from build123d import *

# Parameters (mm, degrees)
SKETCH1_W           = 100
SKETCH1_H           = 20
BOSS_EXTRUDE1_DEPTH = 3
SKETCH2_R           = 4
SKETCH2_R_2         = 1.9
SKETCH2_R_3         = 3
SKETCH2_R_4         = 5
BOSS_EXTRUDE2_DEPTH = 14.25
CHAMFER1_SIZE       = 3
CHAMFER2_SIZE       = 3
CHAMFER3_SIZE       = 3
SKETCH14_R          = 4
SKETCH14_R_2        = 1.8
SKETCH14_R_3        = 5
SKETCH14_R_4        = 6
BOSS_EXTRUDE3_DEPTH = 15
CHAMFER4_SIZE       = 7
CUT_EXTRUDE2_START  = 12
CUT_EXTRUDE2_DEPTH  = 2.4
LPATTERN2_COUNT     = 3
LPATTERN2_PITCH     = 15


with BuildPart() as part:
    # Sketch1 → Boss-Extrude1 (new body)
    with BuildSketch(Plane(origin=(0, 0, 0), x_dir=(1, 0, 0), z_dir=(0, 1, 0))):
        Rectangle(SKETCH1_W, SKETCH1_H)
    extrude(amount=BOSS_EXTRUDE1_DEPTH)

    # Sketch2 → Boss-Extrude2 (add)
    # profile 1 of 3: a face of its own
    with BuildSketch(Plane(origin=(0, 3, 0), x_dir=(1, 0, 0), z_dir=(0, 1, 0))):
        with Locations(Location((-25, 0, 0), (0, 0, 90))):
            Circle(SKETCH2_R)
        with Locations(Location((-25, 0, 0), (0, 0, 90))):
            Circle(SKETCH2_R_2, mode=Mode.SUBTRACT)
    # profile 2 of 3: a face of its own
    with BuildSketch(Plane(origin=(0, 3, 0), x_dir=(1, 0, 0), z_dir=(0, 1, 0))):
        with Locations(Location((-40, 0, 0), (0, 0, 90))):
            Circle(SKETCH2_R_3)
        with Locations(Location((-40, 0, 0), (0, 0, 90))):
            Circle(SKETCH2_R_2, mode=Mode.SUBTRACT)
    # profile 3 of 3: a face of its own
    with BuildSketch(Plane(origin=(0, 3, 0), x_dir=(1, 0, 0), z_dir=(0, 1, 0))):
        with Locations(Location((-10, 0, 0), (0, 0, 90))):
            Circle(SKETCH2_R_4)
        with Locations(Location((-10, 0, 0), (0, 0, 90))):
            Circle(SKETCH2_R_2, mode=Mode.SUBTRACT)
    extrude(amount=BOSS_EXTRUDE2_DEPTH)

    # Chamfer1
    chamfer1_edges = [part.edges().sort_by_distance(p)[0] for p in [
        (-40, 3, 3),
    ]]
    chamfer(chamfer1_edges, length=CHAMFER1_SIZE)

    # Chamfer2
    chamfer2_edges = [part.edges().sort_by_distance(p)[0] for p in [
        (-25, 3, 4),
    ]]
    chamfer(chamfer2_edges, length=CHAMFER2_SIZE)

    # Chamfer3
    chamfer3_edges = [part.edges().sort_by_distance(p)[0] for p in [
        (-10, 3, 5),
    ]]
    chamfer(chamfer3_edges, length=CHAMFER3_SIZE - 0.0001)  # a hair under: the kernel refuses the full size

    # Sketch14 → Boss-Extrude3 (add)
    # profile 1 of 3: a face of its own
    with BuildSketch(Plane(origin=(0, 3, 0), x_dir=(1, 0, 0), z_dir=(0, 1, 0))):
        with Locations(Location((10, 0, 0), (0, 0, 90))):
            Circle(SKETCH14_R)
        with Locations(Location((10, 0, 0), (0, 0, 270))):
            Circle(SKETCH14_R_2, mode=Mode.SUBTRACT)
    # profile 2 of 3: a face of its own
    with BuildSketch(Plane(origin=(0, 3, 0), x_dir=(1, 0, 0), z_dir=(0, 1, 0))):
        with Locations(Location((25, 0, 0), (0, 0, 90))):
            Circle(SKETCH14_R_3)
        with Locations(Location((25, 0, 0), (0, 0, 270))):
            Circle(SKETCH14_R_2, mode=Mode.SUBTRACT)
    # profile 3 of 3: a face of its own
    with BuildSketch(Plane(origin=(0, 3, 0), x_dir=(1, 0, 0), z_dir=(0, 1, 0))):
        with Locations(Location((40, 0, 0), (0, 0, 90))):
            Circle(SKETCH14_R_4)
        with Locations(Location((40, 0, 0), (0, 0, 270))):
            Circle(SKETCH14_R_2, mode=Mode.SUBTRACT)
    extrude(amount=BOSS_EXTRUDE3_DEPTH)

    # Chamfer4
    chamfer4_edges = [part.edges().sort_by_distance(p)[0] for p in [
        (50, 1.5, -10),
    ]]
    chamfer(chamfer4_edges, length=CHAMFER4_SIZE)

    # Sketch16 → Cut-Extrude2 (cut)
    with BuildSketch(Plane(origin=(0, 3, 0), x_dir=(1, 0, 0), z_dir=(0, 1, 0)).offset(CUT_EXTRUDE2_START)):
        Polygon((7.25, -1.58771324), (7.25, -10), (12.75, -10), (12.75, -1.58771324), (12.75, 1.58771324), (10, 3.175426481), (7.25, 1.58771324), align=None)
    cut_extrude2 = extrude(amount=-CUT_EXTRUDE2_DEPTH, mode=Mode.SUBTRACT)

    # LPattern2: Cut-Extrude2 ×3
    with Locations(*[(i * LPATTERN2_PITCH, 0, 0) for i in range(1, LPATTERN2_COUNT)]):
        add(cut_extrude2, mode=Mode.SUBTRACT)


solid = part.part
Check sheet for the modelled part. Datum: model origin and axes. Units: mm. A direction names the side the tool comes from. Coordinates: 2 decimals unless noted, no trailing zeros. Loops run counter-clockwise (first coordinate to the right, second up) from the corner with the lowest first, then second, coordinate; pieces in that order, holes last. Notation, with made-up numbers: (81, -23.75) -> (91, -23.75) arc R19 cw to (91, 11.25) -> close; hole circle Ø9 at (-34, 6.5). An arc over 180 degrees is marked (long way). Write item = value, one per line. Start each with the question number.
1. Material ranges on line 1 (Y direction, x = 27.5, z = 1.75); line 2 (X direction, y = 5.75, z = 2.75); line 3 (Z direction, x = 25, y = 9), recorded low to high.
2. Section check A-A on y = 7. Give the number of separate pieces and of enclosed holes in the cut face, then the cut area to 3 significant figures.
3. Draft check along Y on faces 6 (the flat face through (-1, 0, 0)), 7 (the flat face through (-40, 3, 0)), 8 (the flat face through (24, 15, 2)). Enter one of: released by +Y, released by -Y, zero draft, split by the parting line, or undercut.
4. Section check B-B on x = -10. Record the cut outline in (y, z), then the cut area to 3 significant figures.
5. Tool access check on faces 1 (the flat face through (50, 1, 4)), 2 (the flat face through (27, 18, 0)), 3 (the cylindrical face through (8.243, 7.733, -0.39)), 4 (the flat face through (-38, 17.25, -1)), 5 (the flat face through (8.64, 13.82, -2.39)). Record the directions out of +Z, -Z, +X, -X, +Y, -Y that give a thin tool (end or side, any length) a straight path to the whole face; none if there is none.
6. Section check C-C on x = -25. Record the cut outline in (y, z), then the cut area to 3 significant figures.
7. Depth check by flat-ended pin: P1, Ø3, axis at x = -24, z = -1, coming from the +Y side; P2, Ø2, axis at y = 7.5, z = -6, coming from the +X side; P3, Ø8, axis at x = -5.5, y = 7.5, coming from the -Z side. Enter the tip coordinate at first touch or a pass-through.
Responses:
q1.line_1 = 0 to 12.6, 15 to 18
q1.line_2 = -41.73 to -38.27, -28.24 to -21.76, -14.47 to -5.53, 7.1 to 12.9, 20.82 to 29.18, 34.67 to 45.33
q1.line_3 = -5 to -1.8, 1.8 to 5
q2.separate_pieces = 6
q2.enclosed_holes = 6
q2.area = 334 mm2
q3.face_6 = released by -Y
q3.face_7 = released by +Y
q3.face_8 = undercut
q4.outline = (0, -10) -> (3, -10) -> (3, -8) -> (6, -5) -> (17.25, -5) -> (17.25, -1.9) -> (3, -1.9) -> (3, 1.9) -> (17.25, 1.9) -> (17.25, 5) -> (6, 5) -> (3, 8) -> (3, 10) -> (0, 10) -> close
q4.area = 157 mm2
q5.face_1 = +Z, -Z, +X, +Y, -Y
q5.face_2 = +Z, -Z, +X, -X, +Y
q5.face_3 = +Y
q5.face_4 = +Z, -Z, -X, +Y
q5.face_5 = +Z
q6.outline = (0, -10) -> (3, -10) -> (3, -7) -> (6, -4) -> (17.25, -4) -> (17.25, -1.9) -> (3, -1.9) -> (3, 1.9) -> (17.25, 1.9) -> (17.25, 4) -> (6, 4) -> (3, 7) -> (3, 10) -> (0, 10) -> close
q6.area = 129 mm2
q7.P1 = 17.25
q7.P2 = 43.32
q7.P3 = -6.55
